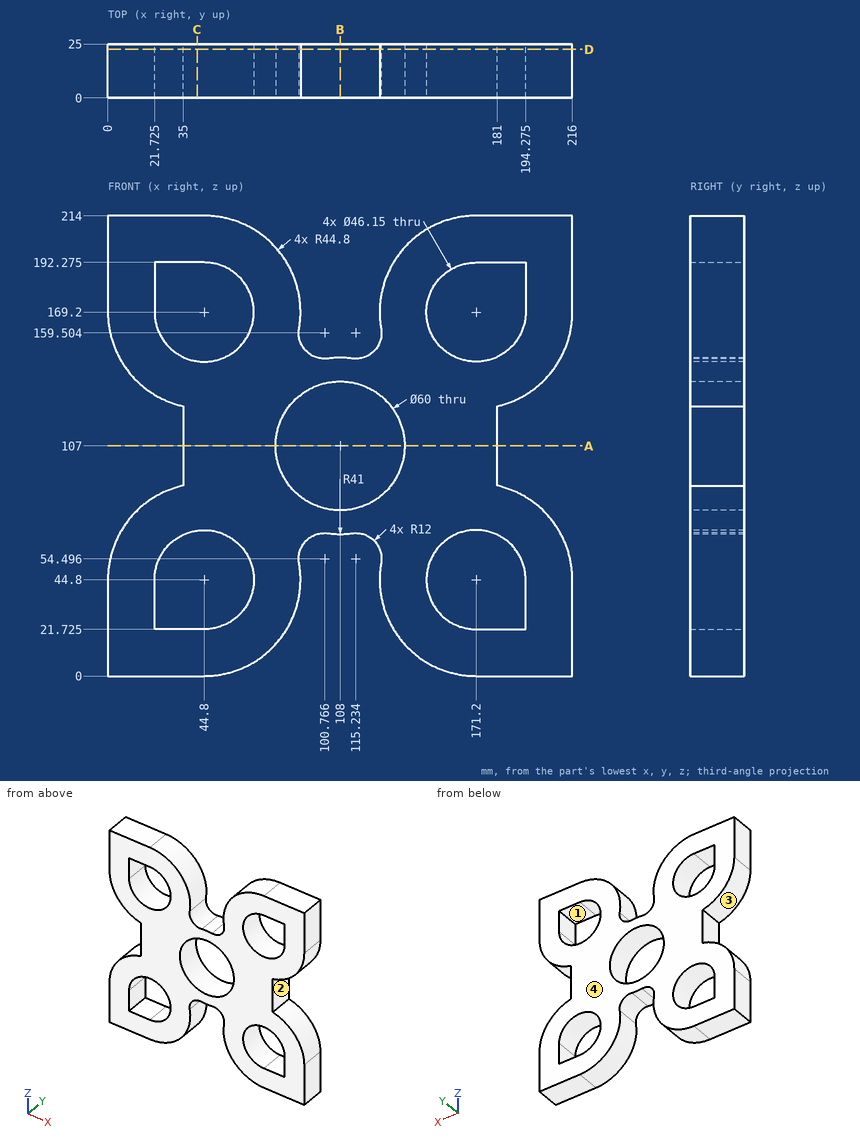
Drawing for the job (mm, zero at the part's lowest x, y, z). A direction names the side the tool comes from. Give positions to 0.01 mm unless a question says otherwise; leave off trailing zeros. Loops run counter-clockwise (first coordinate to the right, second up) from the corner with the lowest first, then second, coordinate; pieces in that order, holes last. Notation, with made-up numbers: (58, 57.5) - (71, 57.5) arc R30 cw to (71, 81.5) - close; hole circle Ø9 at (6, 72). An arc over 180 degrees is marked (long way). Write item = value, one per line. Start each with the question number.
1) Band-saw the part on A-A on z = 107. Give the cut face in (x, y).
2) Probe probe 1 along X at (y, z) = (6.5, 44.8) (1 decimal); probe 2 along Z at (x, y) = (44.8, 7) (1 decimal); probe 3 along Z at (x, y) = (179.5, 13.5) (1 decimal). List the from-to ranges inside material, lowest first. Write a range as from..to.
3) Band-saw the part on D-D on y = 22.5. Count the separate pieces of the cut face and the enclosed holes in it, plus the area to 3 significant figures.
4) Drop flat-ended pins along their axis: pin 1 Ø8 at (y, z) = (11.5, 59) entering from +X; pin 2 Ø3 at (x, z) = (64.5, 46.5) entering from +Y; pin 3 Ø5 at (y, z) = (18, 160) entering from +X; pin 4 Ø12.5 at (y, z) = (10.5, 102.5) entering from +X. Give the stop position or say it passes through.
5) Band-saw the part on B-B on x = 108. Give the cut face in (y, z), plus the area to 3 significant figures.
6) Tool access for the marked faces 1, 2, 3 and 4: list every direction of +Z, -Z, +X, -X, +Y, -Y with a clear straight run to the whole face (end or side of a thin tool).
7) Band-saw the part on C-C on x = 41.5. Give the cut face in (y, z) (1 decimal), plus the area to 3 significant figures.
Final values:
q1.outline = (35, 0) - (78, 0) - (78, 25) - (35, 25) - close; (138, 0) - (181, 0) - (181, 25) - (138, 25) - close
q2.probe_1 = 0..21.7, 67.9..89.6, 126.4..148.1, 194.3..216
q2.probe_2 = 0..21.7, 67.9..146.1, 192.3..214
q2.probe_3 = 0..21.7, 66.3..147.7, 192.3..214
q3.separate_pieces = 1
q3.enclosed_holes = 5
q3.area = 25,600 mm²
q4.pin_1 = 214.82
q4.pin_2 = through
q4.pin_3 = 215.5
q4.pin_4 = 181
q5.outline = (0, 66) - (25, 66) - (25, 77) - (0, 77) - close; (0, 137) - (25, 137) - (25, 148) - (0, 148) - close
q5.area = 550 mm²
q6.face_1 = +Y, -Y
q6.face_2 = +X, +Y, -Y
q6.face_3 = -X, +Y, -Y
q6.face_4 = +Z, -Z, +X, -X, +Y
q7.outline = (0, 0) - (25, 0) - (25, 21.7) - (0, 21.7) - close; (0, 67.6) - (25, 67.6) - (25, 146.4) - (0, 146.4) - close; (0, 192.3) - (25, 192.3) - (25, 214) - (0, 214) - close
q7.area = 3,050 mm²
